Geometry: final body of the model. Coordinates: model frame, mm. A direction names the side the tool comes from. Give positions to 0.01 mm unless a question says otherwise; leave off trailing zeros. Write each loop counter-clockwise with the first axis right and the second up, starting at its lowest first coordinate (ties: lowest second). Pieces come first, ordered by that corner, then holes.
from build123d import *

# Parameters (mm, degrees)
F1_DEPTH = 76.2
F2_DEPTH = 25.4
F3_R     = 20.5394325034
F4_DEPTH = 76.2


with BuildPart() as f1:
    # F0 (on Front) → F1 (new body)
    with BuildSketch(Plane.XZ):
        Polygon((-4.6956427395, 55.8883473277), (-65.5990689993, 55.8883473277), (-65.5990689993, -34.4946607947), (28.3477045596, -34.4946607947), align=None)
    extrude(amount=F1_DEPTH)

    # F0 (on Front) → F2 (join)
    with BuildSketch(Plane.XZ):
        Polygon((-4.6956427395, 55.8883473277), (-65.5990689993, 55.8883473277), (-65.5990689993, -34.4946607947), (28.3477045596, -34.4946607947), align=None)
        Polygon((-65.5990689993, 66.358409822), (-65.5990689993, 55.8883473277), (-4.6956427395, 55.8883473277), (28.3477045596, -34.4946607947), (37.022896111, -34.4946607947), (-4.6956427395, 66.358409822), align=None)
    extrude(amount=-F2_DEPTH)

    # F3 (on face) → F4 (cut)
    with BuildSketch(Plane(origin=(13.8813630625, 0, 5.0749218264), x_dir=(0, 1, 0), z_dir=(0.9392019794, 0, 0.3433651727))):
        with Locations((-37.3390875757, 8.860943839)):
            Circle(F3_R)
    extrude(amount=-F4_DEPTH, mode=Mode.SUBTRACT)


solid = f1.part
Q1. Access query for faces 5 (the flat face through (15.73, -54.5, 0.02)), 6 (the flat face through (-35, -38, 55.888)), 7 (the flat face through (-26, 25.4, 17)). Directions: +Z, -Z, +X, -X, +Y, -Y. A direction counts if a zero-diameter tool reaches every point of the face in a straight line with its end or side. Return the directions, or none.
Filled sheet:
face 5: +Z, +X, -Y
face 6: +Z, +X, -X, -Y
face 7: +Z, -Z, +X, -X, +Y
Q2. Section D-D on x = 24. Output: boundary loops of the cut face in (y, z), plus the area to 3 significant figures.
Filled sheet:
outline: (-76.2, -34.49) - (25.4, -34.49) - (25.4, -3.01) - (0, -3.01) - (0, -22.6) - (-76.2, -22.6) - close
area: 1,710 mm2
Q3. Section C-C on z = 41.5. Output: boundary loops of the cut face in (x, y), plus the area to 3 significant figures.
Filled sheet:
outline: (-65.6, -76.2) - (0.56, -76.2) - (0.56, 0) - (5.59, 0) - (5.59, 25.4) - (-65.6, 25.4) - close
area: 6,850 mm2
Q4. Section A-A on y = -43. Output: boundary loops of the cut face in (x, z).
Filled sheet:
outline: (-65.6, -34.49) - (28.35, -34.49) - (17.62, -5.15) - (-53.95, -31.31) - (-65.6, 0.56) - close; (-65.6, 6.47) - (4.06, 31.94) - (-4.7, 55.89) - (-65.6, 55.89) - close
Q5. Pull-direction query (Y, two-part tool) for faces 1 (the flat face through (-30, -76.2, 11)), 2 (the flat face through (-15, -26, -34.495)), 3 (the cylindrical face through (-24.75, -57.86, 1.35)), 4 (the flat face through (-59.72, -37.63, -15.52)); classes: released by +Y, released by -Y, zero draft, split by the parting line, or undercut.
Filled sheet:
face 1: released by -Y
face 2: zero draft
face 3: undercut
face 4: undercut
Q6. Section B-B on y = 10. Output: boundary loops of the cut face in (x, z).
Filled sheet:
outline: (-65.6, -34.49) - (37.02, -34.49) - (-4.7, 66.36) - (-65.6, 66.36) - close
Q7. Pin query (flat end, axial travel): P1, Ø3, axis at x = -51, y = -6.5, coming from the +Z side; P2, Ø6, axis at x = 10, y = 2.5, coming from the +Z side; P3, Ø4, axis at x = 18, z = 18, coming from the +Y side; P4, Ø3, axis at y = -44.5, z = 34, coming from the +X side. Return the tip coordinate at first contact, or that it passes through.
Filled sheet:
P1: stops at z = 55.89
P2: stops at z = 38.08
P3: passes through
P4: stops at x = 3.85
Q8. Ray query, line 1 along Z through (x, y) = (-37.5, -66); line 2 along Y through (x, z) = (-43, 3.5); line 3 along Y through (x, z) = (-29.5, 60). Return the intervals inside material, ascending.
Filled sheet:
line 1: z = -34.49 to 55.89
line 2: y = -76.2 to -55.71, -18.97 to 25.4
line 3: y = 0 to 25.4
